from build123d import *

# Parameters (mm, degrees)
F2_R = 10


with BuildPart() as f1:
    # F0 (on Right) → F1 (revolve)
    with BuildSketch(Plane.YZ):
        with BuildLine():
            Line((-90.827465, 0), (-37.59887, 0))
            Line((-37.59887, 0), (-37.59887, 45.985954))
            ThreePointArc((-37.59887, 45.985954), (-39.45082, 48.757593), (-42.72019, 48.107275))
            Line((-42.72019, 48.107275), (-90.827465, 0))
        make_face()
    revolve(axis=Axis((0, 0, 38.720641), (0, 0, 1)))

    # F2 (on Right) → F3 (revolve, cut)
    with BuildSketch(Plane.YZ):
        with Locations((-70, 25)):
            Circle(F2_R)
    revolve(axis=Axis((0, 0, 29.182823), (0, 0, 1)), mode=Mode.SUBTRACT)


solid = f1.part
Input: part model. Units: mm. Frame: model coordinates. Coordinates: 2 decimals unless noted, no trailing zeros. Order: outer loops, then holes, each group sorted by start corner. A loop starts at its lowest first (then second) coordinate and runs counter-clockwise, first axis right, second up. Notation, with made-up numbers: M 79.5,40.25 L 96.5,40.25 A21 ccw 96.5,77.25 Z; hole C 4.25,83 d6. An arc over 180 degrees is marked long. Write item = value, one per line. Start each with the question number.
(1) Section D-D on z = 11. Output: boundary loops of the cut face in (x, y).
(2) Pull-direction query (Y, two-part tool) for faces 1 (the cylindrical face through (-22.878, 29.837, 23.315)), 2 (the conical face through (-42.83, 9.511, 46.954)), 3 (the flat face through (1, -39, 0)); classes: released by +Y, released by -Y, zero draft, split by the parting line, or undercut.
(3) Section A-A on x = 0. Output: boundary loops of the cut face in (y, z).
(4) Line query: line 1 along X through (y, z) = (0, 33); line 2 along X through (y, z) = (0, 26.5); line 3 along X through (y, z) = (-38.5, 37). Output: solid intervals per line, ascending. Write a range as [from, to].
(5) Section C-C on z = 43. Output: boundary loops of the cut face in (x, y), and give its area (3 significant figures).
(6) First-contact query: P1, Ø12, axis at x = -38.5, y = 62.5, coming from the +Z side; P2, Ø1, axis at x = -58.5, y = 31, coming from the +Z side; P3, Ø1, axis at x = 55.5, y = -8, coming from the -Z side; P4, Ø1, axis at x = 72.5, y = -33.5, coming from the +Z side. Flat tips, straight axial feed; report the tip coordinate or a pass-through.
Result set:
q1.outline = C 0,0 d159.65; hole C 0,0 d75.2
q2.face_1 = undercut
q2.face_2 = split by the parting line
q2.face_3 = zero draft
q3.outline = M -90.83,0 L -37.6,0 L -37.6,45.99 A3 ccw -42.72,48.11 L -61.16,29.67 A10 cw -74.67,16.16 Z; M 37.6,0 L 90.83,0 L 74.67,16.16 A10 cw 61.16,29.67 L 42.72,48.11 A3 ccw 37.6,45.99 Z
q4.line_1 = [-57.83, -37.6], [37.6, 57.83]
q4.line_2 = [-60.11, -37.6], [37.6, 60.11]
q4.line_3 = [-37.62, 37.62]
q5.outline = C 0,0 d95.65; hole C 0,0 d75.2
q5.area = 2,750 mm²
q6.P1 = 16.16
q6.P2 = 15.97
q6.P3 = 0
q6.P4 = 11.46
